Geometry: final body of the model. Coordinates: model frame, mm. A direction names the side the tool comes from. Round coordinates to 2 decimals unless told otherwise and drop trailing zeros. Loops run counter-clockwise (first coordinate to the right, second up) from the corner with the lowest first, then second, coordinate; pieces in that order, holes last. Notation, with made-up numbers: (-16.5, 36.25) -> (3.5, 36.25) arc R11 ccw to (3.5, 51.25) -> close; hole circle Ø4 at (-11, -5.75). An arc over 180 degrees is marked (long way). Answer in a Markdown table with one row per item.
```python
from build123d import *

# Parameters (mm, degrees)
F1_DEPTH = 5
F2_SIZE  = 2
F3_R     = 0.99999


# Not quite as in the source:
# - a fillet or chamfer is up to 0.001 mm smaller than in the source, because OpenCascade refuses the exact size


with BuildPart() as f1:
    # F0 (on Front) → F1 (new body)
    with BuildSketch(Plane.XZ):
        Polygon((-10.7482137709, -11.0476701237), (-10.7482137709, 3.9523298763), (19.2517862291, 15.9523298763), (18.5090048764, 17.8092832581), (-12.7482137709, 5.3063957992), (-12.7482137709, -9.0476701237), (-23.457470371, -9.0476701237), (-23.457470371, -11.0476701237), align=None)
    extrude(amount=F1_DEPTH)

    # F2
    f2_edges = [f1.edges().sort_by_distance(p)[0] for p in [
        (-12.748214, -2.5, -9.04767),
    ]]
    chamfer(f2_edges, length=F2_SIZE)

    # F3 (radius 1 in the source; OpenCascade refuses exactly that, so slightly less here)
    f3_edges = [f1.edges().sort_by_distance(p)[0] for p in [
        (18.509005, -2.5, 17.809283),
        (19.251786, -2.5, 15.95233),
    ]]
    fillet(f3_edges, radius=F3_R)


solid = f1.part
```
Item 1: Cut plane B-B (z = 0.75). Output: boundary loops of the cut face in (x, y), then the cut area to 3 significant figures.
Answer:
| item | result |
|---|---|
| outline | (-12.75, -5) -> (-10.75, -5) -> (-10.75, 0) -> (-12.75, 0) -> close |
| area | 10.0 mm² |
Item 2: Reachability of faces 1 (the face through (-10.748, -2, -4)), 2 (the face through (-5.5, -5, 6.5)), 3 (the face through (-12.748, -2, -1)) from +Z, -Z, +X, -X, +Y, -Y: full face, straight path, thin tool, end or side. Return the list, or none.
Answer:
| item | result |
|---|---|
| face 1 | -Z, +X, +Y, -Y |
| face 2 | +Z, -Z, +X, -X, -Y |
| face 3 | +Z, -X, +Y, -Y |
Item 3: Pin query (flat end, axial travel): pin 1 Ø1.5 at (y, z) = (-2, 1) entering from -X; pin 2 Ø2.5 at (x, y) = (-20, -2) entering from +Z; pin 3 Ø2 at (x, y) = (8, -4.5) entering from -Z. Return the tip coordinate at first contact, or that it passes through.
Answer:
| item | result |
|---|---|
| pin 1 | stops at x = -12.75 |
| pin 2 | stops at z = -9.05 |
| pin 3 | stops at z = 11.05 |
Item 4: Cut plane C-C (x = 13). Output: boundary loops of the cut face in (y, z), then the cut area to 3 significant figures.
Answer:
| item | result |
|---|---|
| outline | (-5, 13.45) -> (0, 13.45) -> (0, 15.61) -> (-5, 15.61) -> close |
| area | 10.8 mm² |
Item 5: Line query: probe 1 along X at (y, z) = (-4.5, -6.75); probe 2 along Z at (x, y) = (-15.5, -1.85); probe 3 along Z at (x, y) = (13, -2.4). Output: solid intervals per line, ascending. Write a range as [from, to].
Answer:
| item | result |
|---|---|
| probe 1 | x = [-12.75, -10.75] |
| probe 2 | z = [-11.05, -9.05] |
| probe 3 | z = [13.45, 15.61] |
